```python
from build123d import *

# Parameters (mm, degrees)
SKETCH1_R           = 9.75
SKETCH1_R_2         = 3
SKETCH1_R_3         = 1.5
BOSS_EXTRUDE1_DEPTH = 2


with BuildPart() as part:
    # Sketch1 → Boss-Extrude1 (new body)
    with BuildSketch(Plane.XY):
        Circle(SKETCH1_R)
        Circle(SKETCH1_R_2, mode=Mode.SUBTRACT)
        with Locations((0, 7)):
            Circle(SKETCH1_R_3, mode=Mode.SUBTRACT)
        with Locations((4.114496766, 5.663118961)):
            Circle(SKETCH1_R_3, mode=Mode.SUBTRACT)
        with Locations((6.657395614, 2.163118961)):
            Circle(SKETCH1_R_3, mode=Mode.SUBTRACT)
        with Locations((6.657395614, -2.163118961)):
            Circle(SKETCH1_R_3, mode=Mode.SUBTRACT)
        with Locations((4.114496766, -5.663118961)):
            Circle(SKETCH1_R_3, mode=Mode.SUBTRACT)
        with Locations((0, -7)):
            Circle(SKETCH1_R_3, mode=Mode.SUBTRACT)
        with Locations((-4.114496766, -5.663118961)):
            Circle(SKETCH1_R_3, mode=Mode.SUBTRACT)
        with Locations((-6.657395614, -2.163118961)):
            Circle(SKETCH1_R_3, mode=Mode.SUBTRACT)
        with Locations((-6.657395614, 2.163118961)):
            Circle(SKETCH1_R_3, mode=Mode.SUBTRACT)
        with Locations((-4.114496766, 5.663118961)):
            Circle(SKETCH1_R_3, mode=Mode.SUBTRACT)
    extrude(amount=-BOSS_EXTRUDE1_DEPTH)


solid = part.part
```
Geometry: final body of the model. Coordinates: model frame, mm. Round coordinates to 2 decimals unless told otherwise and drop trailing zeros. Order: outer loops, then holes, each group sorted by start corner. A loop starts at its lowest first (then second) coordinate and runs counter-clockwise, first axis right, second up. Notation, with made-up numbers: (-24, 40) -> (24, 40) arc R33 cw to (24, 68) -> close; hole circle Ø1 at (51.25, 88.25). An arc over 180 degrees is marked (long way). Use CSV: the item, a comma, the result in double quotes. Start each with the question number.
1) Section A-A (y = 0). Return the cut outline in (x, z).
2) First-contact query: pin 1 Ø3 at (x, y) = (7.5, -3.5) entering from +Z; pin 2 Ø1.8 at (x, y) = (-6.66, 2.16) entering from +Z. Flat tips, straight axial feed; report the tip coordinate or a pass-through.
3) Draft query along X for faces 1 (the face through (-1.269, 9.667, -0.986)), 2 (the face through (-2.3, 2.3, 0)), 3 (the face through (-3.31, 6.93, -0.99)). Return one class per face: +X half, -X half, draft (parallel to the pull), parting line (faces both ways), or undercut.
4) Section C-C (x = -2.25). Return the cut outline in (y, z).
5) Section D-D (z = -1.25). State how many separate pieces and enclosed holes the cut face has, and give its area (3 significant figures).
6) Material intervals for line 1 along Y through (x, z) = (0, -1.4); line 2 along X through (y, z) = (-6.5, -1.45); line 3 along Y through (x, z) = (8, -1.45), sorted ascending. Write a range as from..to.
7) Section B-B (x = 0). Return the cut outline in (y, z), and give its area (3 significant figures).
Returned:
1,outline,"(-9.75, -2) -> (-3, -2) -> (-3, 0) -> (-9.75, 0) -> close; (3, -2) -> (9.75, -2) -> (9.75, 0) -> (3, 0) -> close"
2,pin 1,"stops at z = 0"
2,pin 2,"passes through"
3,face 1,"parting line"
3,face 2,"draft"
3,face 3,"undercut"
4,outline,"(-9.49, -2) -> (-1.98, -2) -> (-1.98, 0) -> (-9.49, 0) -> close; (1.98, -2) -> (9.49, -2) -> (9.49, 0) -> (1.98, 0) -> close"
5,separate pieces,"1"
5,enclosed holes,"11"
5,area,"200 mm²"
6,line 1,"y = -9.75..-8.5, -5.5..-3, 3..5.5, 8.5..9.75"
6,line 2,"x = -7.27..-5.36, -2.87..-1.41, 1.41..2.87, 5.36..7.27"
6,line 3,"y = -5.57..-2.83, -1.49..1.49, 2.83..5.57"
7,outline,"(-9.75, -2) -> (-8.5, -2) -> (-8.5, 0) -> (-9.75, 0) -> close; (-5.5, -2) -> (-3, -2) -> (-3, 0) -> (-5.5, 0) -> close; (3, -2) -> (5.5, -2) -> (5.5, 0) -> (3, 0) -> close; (8.5, -2) -> (9.75, -2) -> (9.75, 0) -> (8.5, 0) -> close"
7,area,"15.0 mm²"
